Geometry: see drawing. Coordinates: mm, zero at the bounding-box minimum. Coordinates: 2 decimals unless noted, no trailing zeros. Write each loop counter-clockwise with the first axis right and the second up, starting at its lowest first coordinate (ties: lowest second). Pieces come first, ordered by that corner, then holes. Notation, with made-up numbers: (-18, -0.75) - (-1, -0.75) arc R20 ccw to (-1, 34.25) - close; hole circle Ø2 at (70.25, 7). An arc over 180 degrees is marked (long way). Use a Markdown table: item, result. Add a question column.
Q1. Mould query, pull axis Y, two halves, no side actions, for the marked faces 1, 2, 3 and 4. Classes: released by +Y, released by -Y, zero draft, split by the parting line, or undercut.
Q2. Section query B-B (z = 7). Return the cut outline in (x, y).
Q3. Pin query (flat end, axial travel): P1, Ø3, axis at x = 44, y = 14, coming from the +Z side; P2, Ø5, axis at x = 57, y = 22, coming from the -Z side; P3, Ø5, axis at x = 14, y = 14, coming from the +Z side; P4, Ø0.6, axis at y = 17, z = 1, coming from the +X side. Return the tip coordinate at first contact, or that it passes through.
Q4. Section query D-D (z = 1). Return the cut outline in (x, y).
Q5. Material intervals for probe 1 along Y at (x, z) = (44, 5.5); probe 2 along Y at (x, z) = (73.5, 5.5); probe 3 along Z at (x, y) = (80, 4.75), sorted ascending. Write a range as from..to.
Q6. Section query A-A (x = 54). Return the cut outline in (y, z).
Q7. Section query C-C (y = 19.5). Return the cut outline in (x, z), then the cut area to 3 significant figures.
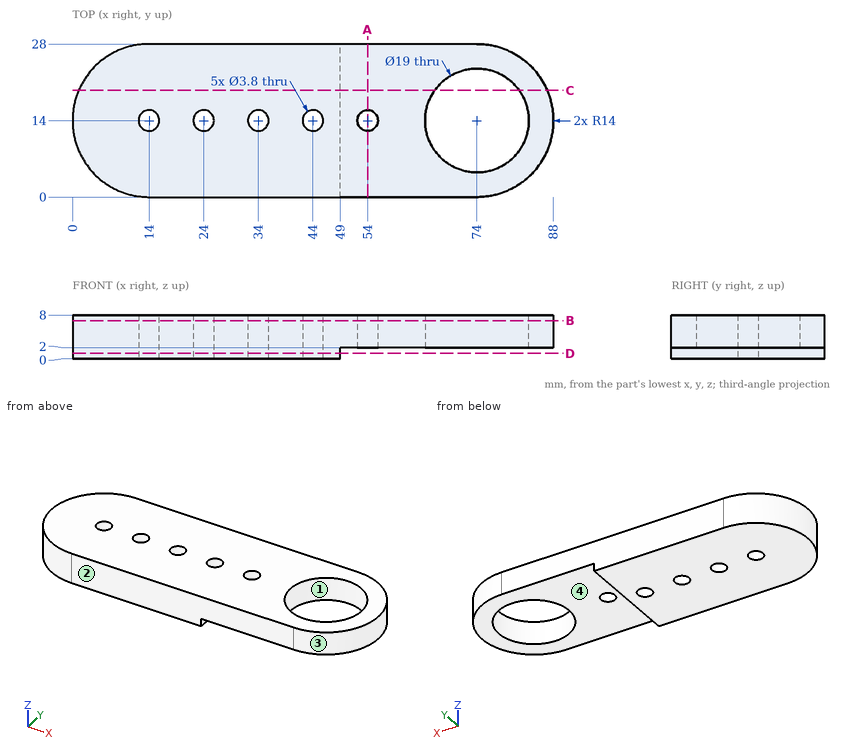
Values follow:
| question | item | result |
|---|---|---|
| 1 | face 1 | undercut |
| 1 | face 2 | released by -Y |
| 1 | face 3 | split by the parting line |
| 1 | face 4 | zero draft |
| 2 | outline | (14, 0) - (74, 0) arc R14 ccw to (74, 28) - (14, 28) arc R14 ccw to start; hole circle Ø3.8 at (14, 14); hole circle Ø3.8 at (24, 14); hole circle Ø3.8 at (34, 14); hole circle Ø3.8 at (44, 14); hole circle Ø3.8 at (54, 14); hole circle Ø19 at (74, 14) |
| 3 | P1 | through |
| 3 | P2 | z = 2 |
| 3 | P3 | z = 8 |
| 3 | P4 | x = 49 |
| 4 | outline | (14, 0) - (49, 0) - (49, 28) - (14, 28) arc R14 ccw to start; hole circle Ø3.8 at (14, 14); hole circle Ø3.8 at (24, 14); hole circle Ø3.8 at (34, 14); hole circle Ø3.8 at (44, 14) |
| 5 | probe 1 | 0..12.1, 15.9..28 |
| 5 | probe 2 | 0..4.51, 23.49..28 |
| 5 | probe 3 | 2..8 |
| 6 | outline | (0, 2) - (12.1, 2) - (12.1, 8) - (0, 8) - close; (15.9, 2) - (28, 2) - (28, 8) - (15.9, 8) - close |
| 7 | outline | (1.13, 0) - (49, 0) - (49, 2) - (66.25, 2) - (66.25, 8) - (1.13, 8) - close; (81.75, 2) - (86.87, 2) - (86.87, 8) - (81.75, 8) - close |
| 7 | area | 517 mm2 |
